Read the model definition and answer for the solid it produces. Units are mm, in the model's axes. A direction names the side the tool comes from. Give positions to 0.01 mm unless a question says otherwise; leave off trailing zeros. Write each loop counter-clockwise with the first axis right and the second up, starting at its lowest first coordinate (ties: lowest second). Pieces come first, ordered by that corner, then holes. Notation, with made-up numbers: (15.5, -5.5) -> (65.5, -5.5) arc R13 cw to (65.5, 4.5) -> close; hole circle Ø11 at (41, -18.75). An arc over 180 degrees is marked (long way). Answer as CSV lines item,"result". Start each with the question number.
1. The part is cut by section C-C, the plane y = 4. Determine the outline of the cut face in (x, z), and give its area (3 significant figures).
2. A tool of negligible diameter and unlimited length cuts with its end or side. For faces 1 (the cylindrical face through (-17, 3.3, -15.57)), 2 (the cylindrical face through (-2.38, 7.24, 10.74)), from which of +Z, -Z, +X, -X, +Y, -Y can it reach the whole face along a straight path? Write none if from no direction.
3. For a pull along Z with two mould halves and no side action, classify faces 3 (the cylindrical face through (-17, 3.3, 15.43)), 4 (the cylindrical face through (-18.92, 6.199, -18.976)), 5 (the cylindrical face through (14, 3.3, -15.57)), 6 (the flat face through (-19.1, 2.7, 19.2)) as pulls with the +Z half, pulls with the -Z half, needs draft (parallel to the pull), parting line crosses it, or undercut.
4. Find the intervals of material crossed by line 1 (Z direction, x = 15.5, y = 1.5); line 2 (X direction, y = 3.25, z = 16), in increasing order.
5. Given pin 1 (2.5 mm diameter, centred on x = 15.5, z = -15.5, fed in from +Y); pin 2 (3.5 mm diameter, centred on x = 15.5, z = 15.5, fed in from +Y), each flat-ended and moving along its own axis, determine where each tip first touches the part or whether it passes through.
6. The part is cut by section B-B, the plane x = -15.5. Determine the outline of the cut face in (y, z), and give its area (3 significant figures).
7. The part is cut by section A-A, the plane z = 15.5. Determine the outline of the cut face in (x, y), and give its area (3 significant figures).
8. The part is cut by section D-D, the plane x = 0. Determine the outline of the cut face in (y, z), and give its area (3 significant figures).
from build123d import *

# Parameters (mm, degrees)
BOSS_EXTRUDE1_DEPTH = 6.5
SKETCH2_R           = 11
BOSS_EXTRUDE2_DEPTH = 2
SKETCH3_R           = 1.5
CUT_EXTRUDE2_DEPTH  = 6.5
SKETCH4_R           = 4.5
CUT_EXTRUDE3_DEPTH  = 8.5
SKETCH5_R           = 5.5
CUT_EXTRUDE4_DEPTH  = 5
FILLET1_R           = 1
FILLET2_R           = 0.5


with BuildPart() as part:
    # Sketch1 → Boss-Extrude1 (new body)
    with BuildSketch(Plane(origin=(0, 0, 0), x_dir=(1, 0, 0), z_dir=(0, 1, 0))):
        Polygon((-21.15, 17.15), (-17.15, 21.15), (17.15, 21.15), (21.15, 17.15), (21.15, -17.15), (17.15, -21.15), (-17.15, -21.15), (-21.15, -17.15), align=None)
    extrude(amount=BOSS_EXTRUDE1_DEPTH)

    # Sketch2 → Boss-Extrude2 (add)
    with BuildSketch(Plane(origin=(0, 6.5, 0), x_dir=(1, 0, 0), z_dir=(0, 1, 0))):
        Circle(SKETCH2_R)
    extrude(amount=BOSS_EXTRUDE2_DEPTH)

    # Sketch3 → Cut-Extrude2 (cut)
    with BuildSketch(Plane(origin=(0, 6.5, 0), x_dir=(1, 0, 0), z_dir=(0, 1, 0))):
        with Locations((-15.5, 15.5)):
            Circle(SKETCH3_R)
        with Locations((15.5, 15.5)):
            Circle(SKETCH3_R)
        with Locations((-15.5, -15.5)):
            Circle(SKETCH3_R)
        with Locations((15.5, -15.5)):
            Circle(SKETCH3_R)
    extrude(amount=-CUT_EXTRUDE2_DEPTH, mode=Mode.SUBTRACT)

    # Sketch4 → Cut-Extrude3 (cut)
    with BuildSketch(Plane(origin=(0, 8.5, 0), x_dir=(1, 0, 0), z_dir=(0, 1, 0))):
        Circle(SKETCH4_R)
    extrude(amount=-CUT_EXTRUDE3_DEPTH, mode=Mode.SUBTRACT)

    # Sketch5 → Cut-Extrude4 (cut)
    with BuildSketch(Plane.XZ):
        Circle(SKETCH5_R)
    extrude(amount=-CUT_EXTRUDE4_DEPTH, mode=Mode.SUBTRACT)

    # Fillet1
    fillet1_edges = [part.edges().sort_by_distance(p)[0] for p in [
        (-21.15, 6.5, 0),
        (-19.15, 6.5, 19.15),
        (0, 6.5, 21.15),
        (19.15, 6.5, 19.15),
        (21.15, 6.5, 0),
        (19.15, 6.5, -19.15),
        (0, 6.5, -21.15),
        (-19.15, 6.5, -19.15),
    ]]
    fillet(fillet1_edges, radius=FILLET1_R)

    # Fillet2
    fillet2_edges = [part.edges().sort_by_distance(p)[0] for p in [
        (-11, 8.5, 0),
    ]]
    fillet(fillet2_edges, radius=FILLET2_R)


solid = part.part
Results found:
1,outline,"(-21.15, -17.15) -> (-17.15, -21.15) -> (17.15, -21.15) -> (21.15, -17.15) -> (21.15, 17.15) -> (17.15, 21.15) -> (-17.15, 21.15) -> (-21.15, 17.15) -> close; hole circle Ø3 at (-15.5, -15.5); hole circle Ø3 at (-15.5, 15.5); hole circle Ø11 at (0, 0); hole circle Ø3 at (15.5, -15.5); hole circle Ø3 at (15.5, 15.5)"
1,area,"1,630 mm²"
2,face 1,"+Y, -Y"
2,face 2,"+Y"
3,face 3,"undercut"
3,face 4,"pulls with the -Z half"
3,face 5,"undercut"
3,face 6,"pulls with the +Z half"
4,line 1,"z = -21.15 to -17, -14 to 14, 17 to 21.15"
4,line 2,"x = -21.15 to -16.91, -14.09 to 14.09, 16.91 to 21.15"
5,pin 1,"passes through"
5,pin 2,"stops at y = 6.5"
6,outline,"(0, -21.15) -> (5.5, -21.15) arc R1 ccw to (6.5, -20.15) -> (6.5, -17) -> (0, -17) -> close; (0, -14) -> (6.5, -14) -> (6.5, 14) -> (0, 14) -> close; (0, 17) -> (6.5, 17) -> (6.5, 20.15) arc R1 ccw to (5.5, 21.15) -> (0, 21.15) -> close"
6,area,"236 mm²"
7,outline,"(-21.15, 0) -> (-17, 0) -> (-17, 6.5) -> (-20.15, 6.5) arc R1 ccw to (-21.15, 5.5) -> close; (-14, 0) -> (14, 0) -> (14, 6.5) -> (-14, 6.5) -> close; (17, 0) -> (21.15, 0) -> (21.15, 5.5) arc R1 ccw to (20.15, 6.5) -> (17, 6.5) -> close"
7,area,"236 mm²"
8,outline,"(0, -21.15) -> (5.5, -21.15) arc R1 ccw to (6.5, -20.15) -> (6.5, -11) -> (8, -11) arc R0.5 ccw to (8.5, -10.5) -> (8.5, -4.5) -> (5, -4.5) -> (5, -5.5) -> (0, -5.5) -> close; (0, 5.5) -> (5, 5.5) -> (5, 4.5) -> (8.5, 4.5) -> (8.5, 10.5) arc R0.5 ccw to (8, 11) -> (6.5, 11) -> (6.5, 20.15) arc R1 ccw to (5.5, 21.15) -> (0, 21.15) -> close"
8,area,"232 mm²"
